Read the model definition and answer for the solid it produces. Units are mm, in the model's axes. Face numbers are marked on the shaded views. A direction names the side the tool comes from. Coordinates: 2 decimals unless noted, no trailing zeros. Order: outer loops, then holes, each group sorted by start corner. A loop starts at its lowest first (then second) coordinate and runs counter-clockwise, first axis right, second up. Notation, with made-up numbers: (56, 2.5) -> (80, 2.5) arc R17 ccw to (80, 17.5) -> close; hole circle Ø7 at (11, -29). An arc over 180 degrees is marked (long way). Use CSV: the item, a comma, the result in double quotes.
```python
from build123d import *

# Parameters (mm, degrees)
BASPROSKE_W           = 8
BASPROSKE_H           = 6
TOOTHCUT_DEPTH        = 12.66190379
TEETHCUTS_COUNT       = 10
TEETHCUTS_ANGLE       = 324
BORSKE_R              = 0.4
BORE_DEPTH            = 50.0000508
CROQUIS1_W            = 5.5
CROQUIS1_H            = 3.7
CORTAR_EXTRUIR1_DEPTH = 6


with BuildPart() as part:
    # BasProSke → Base-Revolve (revolve)
    with BuildSketch(Plane(origin=(0, 0, 0), x_dir=(1, 0, 0), z_dir=(0, 1, 0)), mode=Mode.PRIVATE) as base_revolve_sk:
        with Locations((4, 3)):
            Rectangle(BASPROSKE_W, BASPROSKE_H)
    revolve(base_revolve_sk.sketch.rotate(Axis((-10, 0, 0), (1, 0, 0)), 180), axis=Axis((-10, 0, 0), (1, 0, 0)))

    # TooCutSke → ToothCut (cut, through all)
    with BuildSketch(Plane(origin=(0, 0, 0), x_dir=(0, 0, -1), z_dir=(1, 0, 0))):
        with BuildLine():
            ThreePointArc((0.59278292, 3.701838653), (0, 3.749), (-0.59278292, 3.701838653))
            ThreePointArc((-0.59278292, 3.701838653), (-0.846593509, 4.924114224), (-1.775771316, 5.757784417))
            ThreePointArc((-1.775771316, 5.757784417), (0, 6.0254), (1.775771316, 5.757784417))
            ThreePointArc((1.775771316, 5.757784417), (0.846593509, 4.924114224), (0.59278292, 3.701838653))
        make_face()
    toothcut = extrude(amount=TOOTHCUT_DEPTH, mode=Mode.SUBTRACT)

    # TeethCuts: ToothCut ×10 about axis
    teethcuts_axis = Axis((-10, 0, 0), (1, 0, 0))
    for i in range(1, TEETHCUTS_COUNT):
        add(toothcut.rotate(teethcuts_axis, i * TEETHCUTS_ANGLE / (TEETHCUTS_COUNT - 1)), mode=Mode.SUBTRACT)

    # BorSke → Bore (cut, symmetric)
    with BuildSketch(Plane(origin=(0, 0, 0), x_dir=(0, 0, -1), z_dir=(1, 0, 0))):
        with Locations(Location((0, 0, 0), (0, 0, 180))):
            Circle(BORSKE_R)
    extrude(amount=BORE_DEPTH, both=True, mode=Mode.SUBTRACT)

    # Croquis1 → Cortar-Extruir1 (cut)
    with BuildSketch(Plane(origin=(8, 0, 0), x_dir=(0, 0, -1), z_dir=(1, 0, 0))):
        Rectangle(CROQUIS1_W, CROQUIS1_H)
    extrude(amount=-CORTAR_EXTRUIR1_DEPTH, mode=Mode.SUBTRACT)


solid = part.part
```
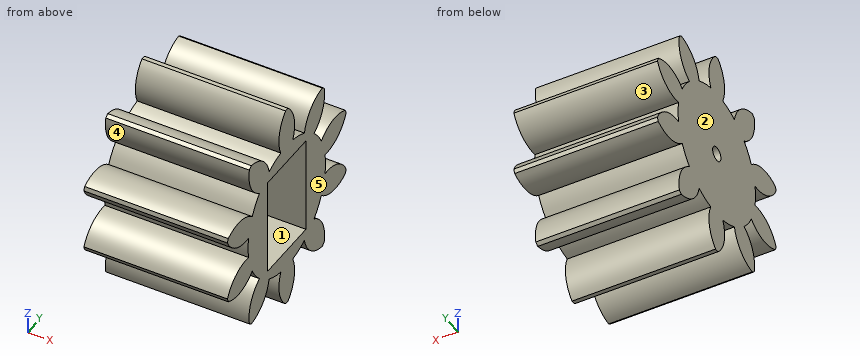
Item 1: A tool of negligible diameter and unlimited length cuts with its end or side. For the marked faces 1 and 2, from which of +Z, -Z, +X, -X, +Y, -Y can it reach the whole face along a straight path? Write none if from no direction.
Return value:
face 1,"+X"
face 2,"+Z, -Z, -X, +Y, -Y"
Item 2: Straight lines are drawn through the part: line 1 along Y through (x, z) = (1.4, 0); line 2 along Z through (x, y) = (6.5, -2.75); line 3 along Y through (x, z) = (5.75, 0). For each, find the intervals that lie inside material, in ascending order.
Return value:
line 1,"y = -3.75 to -0.4, 0.4 to 3.75"
line 2,"z = -4.71 to -2.72, -2.55 to 2.55, 2.72 to 4.71"
line 3,"y = -3.75 to -1.85, 1.85 to 3.75"
Item 3: Find section C-C, the plane z = -4.25. Give the vertices of the cut face in (x, y).
Return value:
outline,"(0, -3.65) -> (8, -3.65) -> (8, -2.16) -> (0, -2.16) -> close; (0, -0.74) -> (8, -0.74) -> (8, 0.74) -> (0, 0.74) -> close; (0, 2.16) -> (8, 2.16) -> (8, 3.65) -> (0, 3.65) -> close"
Item 4: Find section D-D, the plane y = -1.5. Give the vertices of the cut face in (x, z).
Return value:
outline,"(0, -3.44) -> (8, -3.44) -> (8, -2.75) -> (2, -2.75) -> (2, 2.75) -> (8, 2.75) -> (8, 3.44) -> (0, 3.44) -> close"
Item 5: Find section B-B, the plane y = 5.25. Give the vertices of the cut face in (x, z), then the cut area to 3 significant figures.
Return value:
outline,"(0, -2.14) -> (8, -2.14) -> (8, -1.08) -> (0, -1.08) -> close; (0, 1.08) -> (8, 1.08) -> (8, 2.14) -> (0, 2.14) -> close"
area,"17.0 mm^2"
Item 6: The mould has two halves that part along Z. Classify the marked faces 3, 4 and 5: +Z half, -Z half, draft (parallel to the pull), parting line (faces both ways), or undercut.
Return value:
face 3,"undercut"
face 4,"undercut"
face 5,"draft"
Item 7: Find section A-A, the plane z = 0. Give the vertices of the cut face in (x, y).
Return value:
outline,"(0, -3.75) -> (8, -3.75) -> (8, -1.85) -> (2, -1.85) -> (2, -0.4) -> (0, -0.4) -> close; (0, 0.4) -> (2, 0.4) -> (2, 1.85) -> (8, 1.85) -> (8, 3.75) -> (0, 3.75) -> close"
Item 8: Each of these flat-tipped pins is pushed along its axis until it touches: P1, Ø1.8, axis at y = 0.5, z = -0.5, coming from the +X side; P2, Ø1.6, axis at x = 4, z = -0.5, coming from the +Y side; P3, Ø4, axis at x = 5, z = 4, coming from the -Y side. Where does it stop, or does it pass through?
Return value:
P1,"stops at x = 2"
P2,"stops at y = 5.46"
P3,"stops at y = -5.61"
